```python
from build123d import *

# Parameters (mm, degrees)
SKETCH1_W           = 38.1
SKETCH1_H           = 6.35
SKETCH2_R           = 15.875
BOSS_EXTRUDE1_DEPTH = 12.7
CUT_EXTRUDE1_DEPTH  = 14.986
SKETCH10_R          = 4
CUT_EXTRUDE3_DEPTH  = 10
FILLET2_R           = 0.5
SKETCH12_R          = 38.1
SKETCH12_R_2        = 31.75
SKETCH12_R_3        = 2.1828
CUT_EXTRUDE8_DEPTH  = 10
CHAMFER1_SIZE       = 0.4
SKETCH13_R          = 9.09
CUT_EXTRUDE9_DEPTH  = 2.54
CUT_EXTRUDE10_DEPTH = 14.986


with BuildPart() as part:
    # Sketch1 → Revolve1 (revolve)
    with BuildSketch(Plane(origin=(0, 0, 0), x_dir=(1, 0, 0), z_dir=(0, 1, 0))):
        with Locations((19.05, 0)):
            Rectangle(SKETCH1_W, SKETCH1_H)
    revolve(axis=Axis((0, 0, -3.175), (0, 0, 1)))

    # Sketch2 → Boss-Extrude1 (add)
    with BuildSketch(Plane.XY.offset(3.175)):
        Circle(SKETCH2_R)
    extrude(amount=BOSS_EXTRUDE1_DEPTH)

    # Sketch3 → Cut-Extrude1 (cut)
    with BuildSketch(Plane.XY.offset(15.875)):
        with BuildLine():
            Line((-7.813605563, 2.134846154), (-9.769464259, 2.134846154))
            ThreePointArc((-9.769464259, 2.134846154), (-9.999052891, 0.137627323), (-9.824520402, -1.865153846))
            Line((-9.824520402, -1.865153846), (-7.882334751, -1.865153846))
            ThreePointArc((-7.882334751, -1.865153846), (-7.083348537, -3.928889601), (-5.755633784, -5.699357836))
            Line((-5.755633784, -5.699357836), (-6.733563132, -7.393181152))
            ThreePointArc((-6.733563132, -7.393181152), (-5.118715203, -8.590620156), (-3.296989588, -9.440861171))
            Line((-3.296989588, -9.440861171), (-2.325896763, -7.758879059))
            ThreePointArc((-2.325896763, -7.758879059), (-0.139156065, -8.098804578), (2.057971779, -7.83420399))
            Line((2.057971779, -7.83420399), (3.035901127, -9.528027306))
            ThreePointArc((3.035901127, -9.528027306), (4.880337688, -8.728247479), (6.527530814, -7.575707325))
            Line((6.527530814, -7.575707325), (5.556437988, -5.893725213))
            ThreePointArc((5.556437988, -5.893725213), (6.944192472, -4.169914977), (7.813605563, -2.134846154))
            Line((7.813605563, -2.134846154), (9.769464259, -2.134846154))
            ThreePointArc((9.769464259, -2.134846154), (9.999052891, -0.137627323), (9.824520402, 1.865153846))
            Line((9.824520402, 1.865153846), (7.882334751, 1.865153846))
            ThreePointArc((7.882334751, 1.865153846), (7.083348537, 3.928889601), (5.755633784, 5.699357836))
            Line((5.755633784, 5.699357836), (6.733563132, 7.393181152))
            ThreePointArc((6.733563132, 7.393181152), (5.118715203, 8.590620156), (3.296989588, 9.440861171))
            Line((3.296989588, 9.440861171), (2.325896763, 7.758879059))
            ThreePointArc((2.325896763, 7.758879059), (0.139156065, 8.098804578), (-2.057971779, 7.83420399))
            Line((-2.057971779, 7.83420399), (-3.035901127, 9.528027306))
            ThreePointArc((-3.035901127, 9.528027306), (-4.880337688, 8.728247479), (-6.527530814, 7.575707325))
            Line((-6.527530814, 7.575707325), (-5.556437988, 5.893725213))
            ThreePointArc((-5.556437988, 5.893725213), (-6.944192472, 4.169914977), (-7.813605563, 2.134846154))
        make_face()
    extrude(amount=-CUT_EXTRUDE1_DEPTH, mode=Mode.SUBTRACT)

    # Sketch10 → Cut-Extrude3 (cut)
    with BuildSketch(Plane.XY.offset(0.889)):
        Circle(SKETCH10_R)
    extrude(amount=-CUT_EXTRUDE3_DEPTH, mode=Mode.SUBTRACT)

    # Fillet2
    fillet2_edges = [part.edges().sort_by_distance(p)[0] for p in [
        (-15.875, 0, 3.175),
    ]]
    fillet(fillet2_edges, radius=FILLET2_R)

    # Sketch12 → Cut-Extrude8 (cut)
    # profile 1 of 4: a face of its own
    with BuildSketch(Plane(origin=(0, 0, -3.175), x_dir=(-1, 0, 0), z_dir=(0, 0, -1))):
        Circle(SKETCH12_R)
        Circle(SKETCH12_R_2, mode=Mode.SUBTRACT)
    # profile 2 of 4: a face of its own
    with BuildSketch(Plane(origin=(0, 0, -3.175), x_dir=(-1, 0, 0), z_dir=(0, 0, -1))):
        with Locations((0, 23.8125)):
            Circle(SKETCH12_R_3)
    # profile 3 of 4: a face of its own
    with BuildSketch(Plane(origin=(0, 0, -3.175), x_dir=(-1, 0, 0), z_dir=(0, 0, -1))):
        with Locations((-20.622229928, -11.90625)):
            Circle(SKETCH12_R_3)
    # profile 4 of 4: a face of its own
    with BuildSketch(Plane(origin=(0, 0, -3.175), x_dir=(-1, 0, 0), z_dir=(0, 0, -1))):
        with Locations((20.622229928, -11.90625)):
            Circle(SKETCH12_R_3)
    extrude(amount=-CUT_EXTRUDE8_DEPTH, mode=Mode.SUBTRACT)

    # Chamfer1
    chamfer1_edges = [part.edges().sort_by_distance(p)[0] for p in [
        (31.75, 0, 3.175),
        (-15.875, 0, 15.875),
    ]]
    chamfer(chamfer1_edges, length=CHAMFER1_SIZE)

    # Sketch13 → Cut-Extrude9 (cut)
    with BuildSketch(Plane(origin=(0, 0, -3.175), x_dir=(-1, 0, 0), z_dir=(0, 0, -1))):
        Circle(SKETCH13_R)
    extrude(amount=-CUT_EXTRUDE9_DEPTH, mode=Mode.SUBTRACT)

    # Sketch11 → Cut-Extrude10 (cut)
    with BuildSketch(Plane.XY.offset(15.875)):
        with BuildLine():
            Line((-6.78285102, 7.617934894), (-5.807963832, 5.929380754))
            ThreePointArc((-5.807963832, 5.929380754), (-7.117065553, 4.270524315), (-7.964828525, 2.334846154))
            Line((-7.964828525, 2.334846154), (-9.929173855, 2.334846154))
            ThreePointArc((-9.929173855, 2.334846154), (-10.199065112, 0.13809719), (-9.988750652, -2.065153846))
            Line((-9.988750652, -2.065153846), (-8.038976278, -2.065153846))
            ThreePointArc((-8.038976278, -2.065153846), (-7.25691532, -4.028297412), (-6.004450346, -5.730320763))
            Line((-6.004450346, -5.730320763), (-6.986623011, -7.43149372))
            ThreePointArc((-6.986623011, -7.43149372), (-5.219128231, -8.763600887), (-3.205899633, -9.68308874))
            Line((-3.205899633, -9.68308874), (-2.231012445, -7.9945346))
            ThreePointArc((-2.231012445, -7.9945346), (-0.139849768, -8.298821726), (1.96037818, -8.065166917))
            Line((1.96037818, -8.065166917), (2.942550844, -9.766339874))
            ThreePointArc((2.942550844, -9.766339874), (4.979936881, -8.901698077), (6.78285102, -7.617934894))
            Line((6.78285102, -7.617934894), (5.807963832, -5.929380754))
            ThreePointArc((5.807963832, -5.929380754), (7.117065553, -4.270524315), (7.964828525, -2.334846154))
            Line((7.964828525, -2.334846154), (9.929173855, -2.334846154))
            ThreePointArc((9.929173855, -2.334846154), (10.199065112, -0.13809719), (9.988750652, 2.065153846))
            Line((9.988750652, 2.065153846), (8.038976278, 2.065153846))
            ThreePointArc((8.038976278, 2.065153846), (7.25691532, 4.028297412), (6.004450346, 5.730320763))
            Line((6.004450346, 5.730320763), (6.986623011, 7.43149372))
            ThreePointArc((6.986623011, 7.43149372), (5.219128231, 8.763600887), (3.205899633, 9.68308874))
            Line((3.205899633, 9.68308874), (2.231012445, 7.9945346))
            ThreePointArc((2.231012445, 7.9945346), (0.139849768, 8.298821726), (-1.96037818, 8.065166917))
            Line((-1.96037818, 8.065166917), (-2.942550844, 9.766339874))
            ThreePointArc((-2.942550844, 9.766339874), (-4.979936881, 8.901698077), (-6.78285102, 7.617934894))
        make_face()
        with BuildLine():
            Line((-9.769464259, 2.134846154), (-7.813605563, 2.134846154))
            ThreePointArc((-7.813605563, 2.134846154), (-6.944192472, 4.169914977), (-5.556437988, 5.893725213))
            Line((-5.556437988, 5.893725213), (-6.527530814, 7.575707325))
            ThreePointArc((-6.527530814, 7.575707325), (-4.880337688, 8.728247479), (-3.035901127, 9.528027306))
            Line((-3.035901127, 9.528027306), (-2.057971779, 7.83420399))
            ThreePointArc((-2.057971779, 7.83420399), (0.139156065, 8.098804578), (2.325896763, 7.758879059))
            Line((2.325896763, 7.758879059), (3.296989588, 9.440861171))
            ThreePointArc((3.296989588, 9.440861171), (5.118715203, 8.590620156), (6.733563132, 7.393181152))
            Line((6.733563132, 7.393181152), (5.755633784, 5.699357836))
            ThreePointArc((5.755633784, 5.699357836), (7.083348537, 3.928889601), (7.882334751, 1.865153846))
            Line((7.882334751, 1.865153846), (9.824520402, 1.865153846))
            ThreePointArc((9.824520402, 1.865153846), (9.999052891, -0.137627323), (9.769464259, -2.134846154))
            Line((9.769464259, -2.134846154), (7.813605563, -2.134846154))
            ThreePointArc((7.813605563, -2.134846154), (6.944192472, -4.169914977), (5.556437988, -5.893725213))
            Line((5.556437988, -5.893725213), (6.527530814, -7.575707325))
            ThreePointArc((6.527530814, -7.575707325), (4.880337688, -8.728247479), (3.035901127, -9.528027306))
            Line((3.035901127, -9.528027306), (2.057971779, -7.83420399))
            ThreePointArc((2.057971779, -7.83420399), (-0.139156065, -8.098804578), (-2.325896763, -7.758879059))
            Line((-2.325896763, -7.758879059), (-3.296989588, -9.440861171))
            ThreePointArc((-3.296989588, -9.440861171), (-5.118715203, -8.590620156), (-6.733563132, -7.393181152))
            Line((-6.733563132, -7.393181152), (-5.755633784, -5.699357836))
            ThreePointArc((-5.755633784, -5.699357836), (-7.083348537, -3.928889601), (-7.882334751, -1.865153846))
            Line((-7.882334751, -1.865153846), (-9.824520402, -1.865153846))
            ThreePointArc((-9.824520402, -1.865153846), (-9.999052891, 0.137627323), (-9.769464259, 2.134846154))
        make_face(mode=Mode.SUBTRACT)
    extrude(amount=-CUT_EXTRUDE10_DEPTH, mode=Mode.SUBTRACT)


solid = part.part
```
Part model, mm, in its own coordinate system. A direction names the side the tool comes from. Round coordinates to 2 decimals unless told otherwise and drop trailing zeros. Loops run counter-clockwise (first coordinate to the right, second up) from the corner with the lowest first, then second, coordinate; pieces in that order, holes last.
Item 1: Mould opens along X. For faces 1 (the face through (-3.441, -15.497, 9.492)), 2 (the face through (18.606, -12.742, -0.044)), 3 (the face through (0.17, 8.3, 8.49)), 4 (the face through (-7, -7, -3.175)) say: +X half, -X half, draft (parallel to the pull), parting line (faces both ways), or undercut.
Item 2: Cut at A-A, the plane x = 0. State how many separate pieces and enclosed holes the cut face has, then the cut area to 3 significant figures.
Item 3: 3-axis set-ups, long thin cutter, end or side, ignore diameter. For faces 5 (the face through (-6.49, -6.57, 8.49)), 6 (the face through (-2, -4, -0.635)): which of +Z, -Z, +X, -X, +Y, -Y reach the whole face in a straight line?
Item 4: Drop flat-ended pins along their axis: P1, Ø0.6, axis at x = -8.5, z = 12, coming from the -Y side; P2, Ø2, axis at y = 17, z = 12.5, coming from the +X side; P3, Ø7, axis at x = 20.62, y = -11.91, coming from the +Z side (3 decimals); P4, Ø10, axis at y = -22.5, z = 6, coming from the +X side. Give the stop position or say it passes through.
Item 5: Cut at B-B, the plane y = 0. Give the cut face in (x, z) (3 decimals).
Item 6: Drill centre lines: line 1 (Y direction, x = 0, z = -0.75); line 2 (X direction, y = -12, z = 3); line 3 (X direction, y = -9, z = 11.5). Where is each one in solid material? Low to high.
A:
1. face 1: parting line
1. face 2: undercut
1. face 3: undercut
1. face 4: draft
2. separate pieces: 3
2. enclosed holes: 0
2. area: 471 mm2
3. face 5: +Z
3. face 6: -Z
4. P1: stops at y = -13.59
4. P2: passes through
4. P3: stops at z = 3.175
4. P4: stops at x = 25.67
5. outline: (-31.75, -3.175) - (-9.09, -3.175) - (-9.09, -0.635) - (-4, -0.635) - (-4, 0.889) - (-10.2, 0.889) - (-10.2, 15.875) - (-15.475, 15.875) - (-15.875, 15.475) - (-15.875, 3.675) arc R0.5 cw to (-16.375, 3.175) - (-31.35, 3.175) - (-31.75, 2.775) - close; (4, -0.635) - (9.09, -0.635) - (9.09, -3.175) - (31.75, -3.175) - (31.75, 2.775) - (31.35, 3.175) - (16.375, 3.175) arc R0.5 cw to (15.875, 3.675) - (15.875, 15.475) - (15.475, 15.875) - (10.2, 15.875) - (10.2, 0.889) - (4, 0.889) - close
6. line 1: y = -31.75 to -9.09, 9.09 to 21.63, 26 to 31.75
6. line 2: x = -29.15 to -22.8, -18.44 to 18.44, 22.8 to 29.15
6. line 3: x = -13.08 to -4.8, -2.81 to 2.5, 4.8 to 13.08
